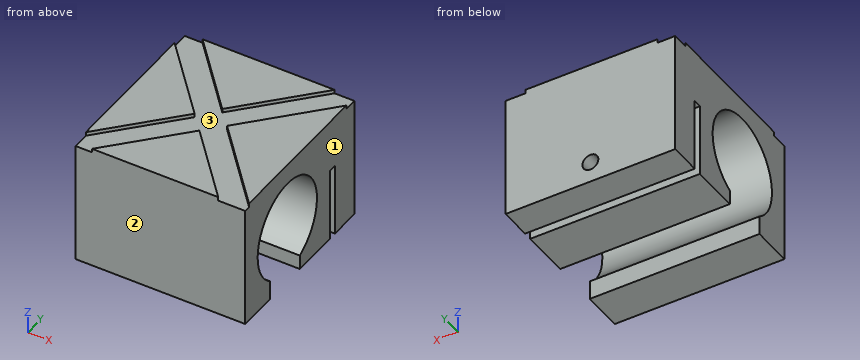
```python
from build123d import *

# Parameters (mm, degrees)
SKETCH1_W           = 67
SKETCH1_H           = 50
BOSS_EXTRUDE1_DEPTH = 70
SKETCH2_R           = 19
CUT_EXTRUDE1_DEPTH  = 70
CUT_EXTRUDE2_DEPTH  = 70
SKETCH4_W           = 29
SKETCH4_H           = 3.3
CUT_EXTRUDE3_DEPTH  = 70
SKETCH5_R           = 3.15
CUT_EXTRUDE4_DEPTH  = 12.5
CUT_EXTRUDE6_DEPTH  = 1.5
CUT_EXTRUDE7_DEPTH  = 1.5


with BuildPart() as part:
    # Sketch1 → Boss-Extrude1 (new body)
    with BuildSketch(Plane(origin=(0, 0, 0), x_dir=(1, 0, 0), z_dir=(0, 1, 0))):
        with Locations((33.5, -25)):
            Rectangle(SKETCH1_W, SKETCH1_H)
    extrude(amount=BOSS_EXTRUDE1_DEPTH)

    # Sketch2 → Cut-Extrude1 (cut)
    with BuildSketch(Plane(origin=(67, 0, 0), x_dir=(0, 0, -1), z_dir=(1, 0, 0))):
        with Locations((-23, 27)):
            Circle(SKETCH2_R)
    extrude(amount=-CUT_EXTRUDE1_DEPTH, mode=Mode.SUBTRACT)

    # Sketch3 → Cut-Extrude2 (cut)
    with BuildSketch(Plane(origin=(67, 0, 0), x_dir=(0, 0, -1), z_dir=(1, 0, 0))):
        Polygon((0, 25.5), (0, 35), (-5.76631206, 35), (-4, 27), (-7.506256635, 16.002549544), (0, 16), align=None)
    extrude(amount=-CUT_EXTRUDE2_DEPTH, mode=Mode.SUBTRACT)

    # Sketch4 → Cut-Extrude3 (cut)
    with BuildSketch(Plane(origin=(67, 0, 0), x_dir=(0, 0, -1), z_dir=(1, 0, 0))):
        with Locations((-14.5, 55.85)):
            Rectangle(SKETCH4_W, SKETCH4_H)
    extrude(amount=-CUT_EXTRUDE3_DEPTH, mode=Mode.SUBTRACT)

    # Sketch5 → Cut-Extrude4 (cut)
    with BuildSketch(Plane(origin=(0, 70, 0), x_dir=(1, 0, 0), z_dir=(0, 1, 0))):
        with Locations(Location((33.5, -8.3, 0), (0, 0, 270))):
            Circle(SKETCH5_R)
    extrude(amount=-CUT_EXTRUDE4_DEPTH, mode=Mode.SUBTRACT)

    # Sketch6 → Cut-Extrude6 (cut)
    with BuildSketch(Plane.XY.offset(50)):
        Polygon((0, 63.425021167), (56.359161664, 0), (67, 0), (67, 2.477681398), (7, 70), (0, 70), align=None)
    extrude(amount=-CUT_EXTRUDE6_DEPTH, mode=Mode.SUBTRACT)

    # Sketch7 → Cut-Extrude7 (cut)
    with BuildSketch(Plane.XY.offset(50)):
        Polygon((0, 6.564878252), (59.179714273, 70), (67, 70), (67, 64.848472441), (6.501746598, 0), (0, 0), align=None)
    extrude(amount=-CUT_EXTRUDE7_DEPTH, mode=Mode.SUBTRACT)


solid = part.part
```
The listing builds one solid part. Answer for the finished solid, in the listing's coordinates (mm). Face numbers are marked on the shaded views. Coordinates: 2 decimals unless noted, no trailing zeros. Write each loop counter-clockwise with the first axis right and the second up, starting at its lowest first coordinate (ties: lowest second). Pieces come first, ordered by that corner, then holes. Notation, with made-up numbers: M -4,17.25 L 41,17.25 A15 ccw 41,29.25 Z; hole C -36.5,70 d5. An arc over 180 degrees is marked long. Use a Markdown table: item, result. Add a question column.
1. Straight lines are drawn through the part: line 1 along Y through (x, z) = (44.5, 3); line 2 along Y through (x, z) = (21, 23); line 3 along X through (y, z) = (63.25, 8.3). For each, find the intervals that lie inside material, in ascending order. Write a range as [from, to].
2. Given P1, Ø4, axis at x = 33.5, z = 8.3, coming from the +Y side; P2, Ø1, axis at x = 32, y = 55.5, coming from the -Z side, each flat-ended and moving along its own axis, determine where each tip first touches the part or whether it passes through.
3. Section B-B (y = 10) is taken. Give the vertices of the cut face in (x, z), plus the area to 3 significant figures.
4. Section C-C (x = 33.5) is taken. Give the vertices of the cut face in (y, z).
5. Section A-A (z = 23) is taken. Give the vertices of the cut face in (x, y).
6. For a pull along Y with two mould halves and no side action, classify the marked faces 1, 2 and 3 as +Y half, -Y half, draft (parallel to the pull), parting line (faces both ways), or undercut.
7. Section D-D (z = 40) is taken. Give the vertices of the cut face in (x, y), plus the area to 3 significant figures.
Data:
| question | item | result |
|---|---|---|
| 1 | line 1 | y = [0, 16], [35, 54.2], [57.5, 70] |
| 1 | line 2 | y = [0, 8], [46, 54.2], [57.5, 70] |
| 1 | line 3 | x = [0, 30.35], [36.65, 67] |
| 2 | P1 | stops at y = 54.2 |
| 2 | P2 | stops at z = 29 |
| 3 | outline | M 0,0 L 67,0 L 67,14.51 L 0,14.51 Z; M 0,31.49 L 67,31.49 L 67,50 L 60.32,50 L 60.32,48.5 L 47.47,48.5 L 47.47,50 L 15.83,50 L 15.83,48.5 L 3.2,48.5 L 3.2,50 L 0,50 Z |
| 3 | area | 2,170 mm2 |
| 4 | outline | M 0,0 L 16,0 L 16,7.51 A19 cw long 35,5.77 L 35,0 L 54.2,0 L 54.2,29 L 57.5,29 L 57.5,11.45 L 70,11.45 L 70,50 L 42.47,50 L 42.47,48.5 L 25.73,48.5 L 25.73,50 L 0,50 Z; M 57.5,0 L 70,0 L 70,5.15 L 57.5,5.15 Z |
| 5 | outline | M 0,0 L 67,0 L 67,8 L 0,8 Z; M 0,46 L 67,46 L 67,54.2 L 0,54.2 Z; M 0,57.5 L 67,57.5 L 67,70 L 0,70 Z |
| 6 | face 1 | draft |
| 6 | face 2 | -Y half |
| 6 | face 3 | undercut |
| 7 | outline | M 0,0 L 67,0 L 67,18.51 L 0,18.51 Z; M 0,35.49 L 67,35.49 L 67,70 L 0,70 Z |
| 7 | area | 3,550 mm2 |
